The listing builds one solid part. Answer for the finished solid, in the listing's coordinates (mm). Face numbers are marked on the shaded views. A direction names the side the tool comes from. Round coordinates to 2 decimals unless told otherwise and drop trailing zeros. Write each loop counter-clockwise with the first axis right and the second up, starting at its lowest first coordinate (ties: lowest second). Pieces come first, ordered by that corner, then holes.
(1) A cutting plane is placed at B-B, the plane y = 11. Give the vertices of the cut face in (x, z), and give its area (3 significant figures).
(2) A cutting plane is placed at A-A, the plane z = -27. Give the vertices of the cut face in (x, y).
(3) A cutting plane is placed at C-C, the plane z = -4. Give the vertices of the cut face in (x, y), and give its area (3 significant figures).
(4) A cutting plane is placed at D-D, the plane x = 6. Give the vertices of the cut face in (y, z).
(5) For the marked faces 1, 2, 3, 4 and 5, determine the directions among +Z, -Z, +X, -X, +Y, -Y from which every point of the face is accessible in a straight line to the end or side of a thin tool.
(6) Each of these flat-tipped pins is pushed along its axis until it touches: pin 1 Ø6 at (y, z) = (30, -36) entering from +X; pin 2 Ø12 at (y, z) = (47.5, -48.5) entering from -X; pin 3 Ø8.5 at (x, z) = (-36, -15.5) entering from +Y; pin 4 Ø11 at (x, z) = (37.21, -27) entering from +Y. Where does it stop, or does it pass through?
(7) The mould has two halves that part along Z. Classify the marked faces 6, 7 and 8: +Z half, -Z half, draft (parallel to the pull), parting line (faces both ways), or undercut.
(8) Find the intervals of material crossed by probe 1 along Y at (x, z) = (40.5, -33.5); probe 2 along X at (y, z) = (23.5, -26); probe 3 along X at (y, z) = (45.5, -12.5), in increasing order.
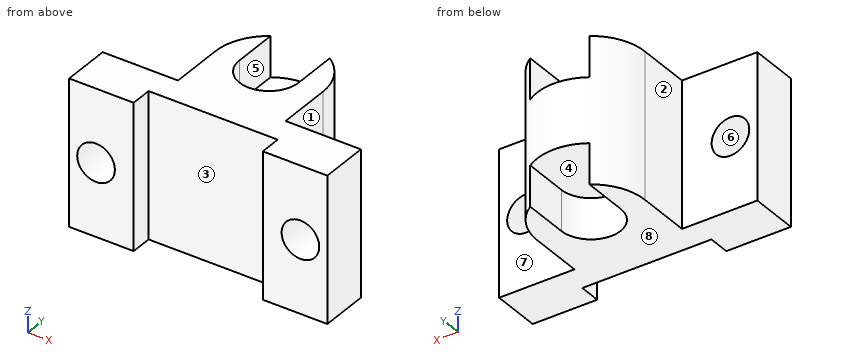
from build123d import *

# Parameters (mm, degrees)
BOSS_EXTRUDE1_DEPTH = 54
SKETCH2_R           = 7
CUT_EXTRUDE1_DEPTH  = 54
CUT_EXTRUDE2_DEPTH  = 15
CUT_EXTRUDE3_START  = -15
CUT_EXTRUDE3_DEPTH  = 15


with BuildPart() as part:
    # Sketch1 → Boss-Extrude1 (new body)
    with BuildSketch(Plane.XY):
        with BuildLine():
            Line((-48.791461113, 0), (-24.791461113, 0))
            Line((-24.791461113, 0), (-24.791461113, 8))
            Line((-24.791461113, 8), (23.208538887, 8))
            Line((23.208538887, 8), (23.208538887, 0))
            Line((23.208538887, 0), (47.208538887, 0))
            Line((47.208538887, 0), (47.208538887, 18))
            Line((47.208538887, 18), (19.208538887, 18))
            Line((19.208538887, 18), (19.208538887, 38))
            ThreePointArc((19.208538887, 38), (-0.791461113, 58), (-20.791461113, 38))
            Line((-20.791461113, 38), (-20.791461113, 18))
            Line((-20.791461113, 18), (-48.791461113, 18))
            Line((-48.791461113, 18), (-48.791461113, 0))
        make_face()
    extrude(amount=-BOSS_EXTRUDE1_DEPTH)

    # Sketch2 → Cut-Extrude1 (cut)
    with BuildSketch(Plane(origin=(0, 18, 0), x_dir=(1, 0, 0), z_dir=(0, 1, 0))):
        with Locations(Location((37.208538887, 27, 0), (0, 0, 180))):
            Circle(SKETCH2_R)
        with Locations(Location((-38.791461113, 27, 0), (0, 0, 180))):
            Circle(SKETCH2_R)
    extrude(amount=-CUT_EXTRUDE1_DEPTH, mode=Mode.SUBTRACT)

    # Sketch3 → Cut-Extrude2 (cut)
    with BuildSketch(Plane.XY):
        with BuildLine():
            Line((10.208538887, 58), (10.208538887, 38))
            ThreePointArc((10.208538887, 38), (-0.791461113, 27), (-11.791461113, 38))
            Line((-11.791461113, 38), (-11.791461113, 58))
            ThreePointArc((-11.791461113, 58), (-0.791461113, 69), (10.208538887, 58))
        make_face()
    extrude(amount=-CUT_EXTRUDE2_DEPTH, mode=Mode.SUBTRACT)

    # Sketch4 → Cut-Extrude3 (cut)
    with BuildSketch(Plane(origin=(0, 0, -54), x_dir=(-1, 0, 0), z_dir=(0, 0, -1)).offset(CUT_EXTRUDE3_START)):
        with BuildLine():
            Line((11.791461113, 58), (11.791461113, 38))
            ThreePointArc((11.791461113, 38), (0.791461113, 27), (-10.208538887, 38))
            Line((-10.208538887, 38), (-10.208538887, 58))
            ThreePointArc((-10.208538887, 58), (0.791461113, 69), (11.791461113, 58))
        make_face()
    extrude(amount=CUT_EXTRUDE3_DEPTH, mode=Mode.SUBTRACT)


solid = part.part
Solutions:
1. outline: (-48.79, -54) - (47.21, -54) - (47.21, 0) - (-48.79, 0) - close; hole circle Ø14 at (-38.79, -27); hole circle Ø14 at (37.21, -27)
1. area: 4,880 mm2
2. outline: (-48.79, 0) - (-45.79, 0) - (-45.79, 18) - (-48.79, 18) - close; (-31.79, 0) - (-24.79, 0) - (-24.79, 8) - (23.21, 8) - (23.21, 0) - (30.21, 0) - (30.21, 18) - (19.21, 18) - (19.21, 38) arc R20 ccw to (-20.79, 38) - (-20.79, 18) - (-31.79, 18) - close; (44.21, 0) - (47.21, 0) - (47.21, 18) - (44.21, 18) - close
3. outline: (-48.79, 0) - (-24.79, 0) - (-24.79, 8) - (23.21, 8) - (23.21, 0) - (47.21, 0) - (47.21, 18) - (19.21, 18) - (19.21, 38) arc R20 ccw to (10.21, 54.7) - (10.21, 38) arc R11 cw to (-11.79, 38) - (-11.79, 54.7) arc R20 ccw to (-20.79, 38) - (-20.79, 18) - (-48.79, 18) - close
3. area: 2,170 mm2
4. outline: (8, -54) - (29.35, -54) - (29.35, -39) - (56.81, -39) - (56.81, -15) - (29.35, -15) - (29.35, 0) - (8, 0) - close
5. face 1: +Z, -Z, +X, +Y
5. face 2: +Z, -Z, -X, +Y
5. face 3: +Z, -Z, -Y
5. face 4: -Z, +Y
5. face 5: +Z, +Y
6. pin 1: stops at x = 19.21
6. pin 2: stops at x = -20.48
6. pin 3: stops at y = 18
6. pin 4: passes through
7. face 6: undercut
7. face 7: draft
7. face 8: -Z half
8. probe 1: y = 0 to 18
8. probe 2: x = -20.79 to 19.21
8. probe 3: x = -19.33 to -11.79, 10.21 to 17.75
